Autodesk Inventor part; units mm, degrees
ref_plane "YZ Plane" through (0, 0, 0) normal (1, 0, 0) x (0, 1, 0)
ref_plane "XZ Plane" through (0, 0, 0) normal (0, 1, 0) x (-1, 0, 0)
ref_plane "XY Plane" through (0, 0, 0) normal (0, 0, 1) x (1, 0, 0)
sketch "Sketch1" plane through (0, 0, 0) normal (0, 0, 1) x (1, 0, 0)
  line L0 (0, 12.6) -> (150, 12.6)
  arc A0 (150, -12.6) -> (150, 12.6) centre (150, 0) ccw
  line L1 (150, -12.6) -> (0, -12.6)
  arc A1 (0, 12.6) -> (0, -12.6) centre (0, 0) ccw
  circle A2 centre (0, 0) radius 7.5
  circle A3 centre (150, 0) radius 4.25
  dimension "d0" = 150
  dimension "d2" = 12.6
  dimension "d3" = 15
  dimension "d4" = 8.5
extrude "Extrusion1" add sketch "Sketch1" along normal blind 21.1
sketch "Sketch2" plane through (0, 0, 21.1) normal (0, 0, 1) x (1, 0, 0)
  circle A0 centre (0, 0) radius 7.5
  arc A1 (0, 12.6) -> (0, -12.6) centre (0, 0) ccw
  circle A2 centre (0, 0) radius 11
  dimension "d7" = 22
extrude "Extrusion2" cut sketch "Sketch2" against normal blind 7
sketch "Sketch4" plane through (0, 0, 21.1) normal (0, 0, 1) x (1, 0, 0)
  circle A0 centre (0, 0) radius 11
  circle A1 centre (20, 0) radius 1.75
  circle A2 centre (40, 0) radius 1.75
  dimension "d16" = 20
  dimension "d17" = 40
  dimension "d23" = 3.5
extrude "Extrusion3" cut sketch "Sketch4" against normal through all contours A1 | A2
sketch "Sketch5" plane through (0, 0, 21.1) normal (0, 0, 1) x (1, 0, 0)
  circle A0 centre (20, 0) radius 1.75
  circle A1 centre (40, 0) radius 1.75
  circle A2 centre (40, 0) radius 3
  circle A3 centre (20, 0) radius 3
  dimension "d28" = 6
extrude "Extrusion4" cut sketch "Sketch5" against normal blind 3
sketch "Sketch6" plane through (0, 0, 21.1) normal (0, 0, 1) x (1, 0, 0)
  line L0 (150, 12.6) -> (0, 12.6)
  arc A0 (0, 12.6) -> (0, -12.6) centre (0, 0) ccw
  line L1 (0, -12.6) -> (150, -12.6)
  arc A1 (12.1445, 12.6) -> (12.1445, -12.6) centre (0, 0) ccw
  dimension "d24" = 35
extrude "Extrusion5" add sketch "Sketch6" against normal up to surface (21.1 mm away)
fillet "Fillet1" radius 3.5 1 edges at (-7.5, 0, 14.1)
sketch "Sketch8" plane through (0, 0, 21.1) normal (0, 0, 1) x (1, 0, 0)
  circle A0 centre (150, 0) radius 7
  line L0 (150, 12.6) -> (12.1445, 12.6)
  arc A1 (12.1445, 12.6) -> (12.1445, -12.6) centre (0, 0) ccw
  line L1 (12.1445, -12.6) -> (150, -12.6)
  line L2 (100, 12.6) -> (100, 5.75)
  line L3 (100, 5.75) -> (50, 5.75)
  line L4 (50, 5.75) -> (50, -5.75)
  line L5 (50, -5.75) -> (100, -5.75)
  line L6 (100, -5.75) -> (100, -12.6)
  circle A2 centre (40, 0) radius 3
  circle A3 centre (20, 0) radius 3
  circle A4 centre (0, 0) radius 11
  circle A5 centre (150, 0) radius 4.25
  line L7 (150, 12.6) -> (12.1445, 12.6)
  arc A6 (12.1445, 12.6) -> (12.1445, -12.6) centre (0, 0) ccw
  line L8 (12.1445, -12.6) -> (150, -12.6)
  arc A7 (150, -12.6) -> (150, 12.6) centre (150, 0) ccw
  dimension "d35" = 50
  dimension "d36" = 50
  dimension "d37" = 11.5
extrude "Extrusion7" cut sketch "Sketch8" against normal through all contours L2 L3 L4 L5 L6 L1 A1 L0 | A2 | A3 | A4
sketch "Sketch9" plane through (50, -5.75, 21.1) normal (0, -1, 0) x (1, 0, 0)
  line L0 (0, 0) -> (0, -21.1)
  line L1 (4.5, -6.55) -> (12.5, -6.55) construction
  line L2 (12.5, -6.55) -> (12.5, -14.55) construction
  line L3 (12.5, -14.55) -> (4.5, -14.55) construction
  line L4 (4.5, -14.55) -> (4.5, -6.55) construction
  line L5 (12.5, -14.55) -> (20.5, -14.55) construction
  line L6 (20.5, -14.55) -> (20.5, -6.55) construction
  line L7 (20.5, -6.55) -> (12.5, -6.55) construction
  line L8 (12.5, -6.55) -> (12.5, -14.55) construction
  circle A0 centre (4.5, -14.55) radius 1.75
  circle A1 centre (4, -6.55) radius 1.75
  circle A2 centre (11.5, -14.55) radius 1.75
  circle A3 centre (11, -6.55) radius 1.75
  circle A4 centre (18.5, -14.55) radius 1.75
  circle A5 centre (18, -6.55) radius 1.75
  line L9 (29.5, -6.55) -> (37.5, -6.55) construction
  line L10 (37.5, -6.55) -> (37.5, -14.55) construction
  line L11 (37.5, -14.55) -> (29.5, -14.55) construction
  line L12 (29.5, -14.55) -> (29.5, -6.55) construction
  line L13 (37.5, -14.55) -> (45.5, -14.55) construction
  line L14 (45.5, -14.55) -> (45.5, -6.55) construction
  line L15 (45.5, -6.55) -> (37.5, -6.55) construction
  line L16 (37.5, -6.55) -> (37.5, -14.55) construction
  circle A6 centre (29.5, -6.55) radius 1.75
  circle A7 centre (29, -14.55) radius 1.75
  circle A8 centre (36.5, -6.55) radius 1.75
  circle A9 centre (36, -14.55) radius 1.75
  circle A10 centre (43.5, -6.55) radius 1.75
  circle A11 centre (43, -14.55) radius 1.75
  point P0 (-50, -21.1)
  point P1 (0, -10.55)
  point P2 (12.5, -10.55)
  point P3 (12.5, -10.55)
  point P4 (37.5, -10.55)
  dimension "d40" = 12.5
  dimension "d41" = 8
  dimension "d42" = 0.5
  dimension "d43" = 1
  dimension "d44" = 1.5
  dimension "d45" = 2
  dimension "d46" = 2.5
  dimension "d47" = 3.5
  dimension "d48" = 25
  dimension "d49" = 0.5
  dimension "d50" = 1
  dimension "d51" = 1.5
  dimension "d52" = 2
  dimension "d53" = 2.5
extrude "Extrusion8" cut sketch "Sketch9" against normal through all
sketch "Sketch10" plane through (0, 0, 0) normal (0, 0, -1) x (-1, 0, 0)
  circle A0 centre (-150, 0) radius 4.25
  line L0 (-157.5056, 0) -> (-153.7528, 6.5)
  line L1 (-153.7528, 6.5) -> (-146.2472, 6.5)
  line L2 (-146.2472, 6.5) -> (-142.4944, 0)
  line L3 (-142.4944, 0) -> (-146.2472, -6.5)
  line L4 (-146.2472, -6.5) -> (-153.7528, -6.5)
  line L5 (-153.7528, -6.5) -> (-157.5056, 0)
  point P0 (0, 0)
  dimension "d56" = 13
extrude "Extrusion9" cut sketch "Sketch10" against normal blind 8
properties part number "thin arm2_2"
Build history of the part. All positions in model axes, mm. A direction names the side the tool comes from. Coordinates: 2 decimals unless noted, no trailing zeros. Order: outer loops, then holes, each group sorted by start corner. A loop starts at its lowest first (then second) coordinate and runs counter-clockwise, first axis right, second up. Notation, with made-up numbers: (-19, 61.25) - (3, 61.25) arc R24 cw to (3, 76.25) - close; hole circle Ø4 at (40.25, 47.25). An arc over 180 degrees is marked (long way). Write each question's results on one line, items separated by ' | '. Start each with the question number.
Item 1: Tool access for faces 4 (the face through (75, 5.75, 11)), 5 (the face through (150, -6.5, 4)), 6 (the face through (75, -5.75, 11)): list every direction of +Z, -Z, +X, -X, +Y, -Y with a clear straight run to the whole face (end or side of a thin tool).
Item 2: Band-saw the part on C-C on x = 93. Write the cut outline in (y, z).
Item 3: Flat gauge pins, fed straight in: pin 1 (4.5 mm diameter, centred on x = 54, z = 14.55, fed in from -Y); pin 2 (5.5 mm diameter, centred on x = 54.5, z = 6.55, fed in from +Y); pin 3 (1 mm diameter, centred on y = 1, z = 14.5, fed in from +X). Where does each tip first touch, or does it go through?
Item 4: Band-saw the part on A-A on z = 14.55. State how many separate pieces and enclosed holes the cut face has, and give its area (3 significant figures).
Item 5: Mould opens along Y. For faces 1 (the face through (162.597, 0.277, 10.402)), 2 (the face through (100, 9, 11)), 3 (the face through (155.66, 3.2, 3.94)) say: released by +Y, released by -Y, zero draft, split by the parting line, or undercut.
Item 6: Wall check: probe 1 along Z at (x, y) = (68, 2.5); probe 2 along Z at (x, y) = (93, -1); probe 3 along Y at (x, z) = (155.5, 5.75). Give the ranges that are in metal, low to high. Write a range as [from, to].
Numbers:
1) face 4: +Z, -Z, -X, +Y | face 5: -Z | face 6: +Z, -Z, -X, -Y
2) outline: (-5.75, 0) - (5.75, 0) - (5.75, 4.8) - (-5.75, 4.8) - close; (-5.75, 8.3) - (5.75, 8.3) - (5.75, 12.87) - (-5.75, 12.87) - close; (-5.75, 16.23) - (5.75, 16.23) - (5.75, 21.1) - (-5.75, 21.1) - close
3) pin 1: y = -5.75 | pin 2: y = 5.75 | pin 3: x = 162.59
4) separate pieces: 7 | enclosed holes: 1 | area: 1,790 mm^2
5) face 1: split by the parting line | face 2: zero draft | face 3: undercut
6) probe 1: [0, 4.87], [8.23, 12.8], [16.3, 21.1] | probe 2: [0, 4.8], [8.3, 12.87], [16.23, 21.1] | probe 3: [-11.34, -3.47], [3.47, 11.34]
